Autodesk Inventor part; units mm, degrees
ref_plane "YZ Plane" through (0, 0, 0) normal (1, 0, 0) x (0, 1, 0)
ref_plane "XZ Plane" through (0, 0, 0) normal (0, 1, 0) x (-1, 0, 0)
ref_plane "XY Plane" through (0, 0, 0) normal (0, 0, 1) x (1, 0, 0)
sketch "Sketch1" plane through (0, 0, 0) normal (0, 1, 0) x (-1, 0, 0)
  line L0 (7.056, 3.3) -> (-24.7, 3.3)
  line L1 (-24.7, 3.3) -> (-24.7, 5.5)
  line L2 (-24.7, 5.5) -> (-20.7, 5.5)
  line L3 (-20.7, 5.5) -> (-20.2, 5)
  line L4 (-20.2, 5) -> (20.2, 5)
  line L5 (20.2, 5) -> (20.7, 5.5)
  line L6 (20.7, 5.5) -> (24.7, 5.5)
  line L7 (24.7, 5.5) -> (24.7, 3.3)
  line L8 (24.7, 3.3) -> (7.056, 3.3)
  line L9 (0, -1.1) -> (0, 6.6) construction
  line L10 (-34.58, 0) -> (34.58, 0) construction
  point P0 (0, 0)
  dimension "d0" = 3.3
  dimension "d1" = 40.4
  dimension "d2" = 49.4
  dimension "d3" = 0.5
  dimension "d4" = 5
revolve "Revolution1" add sketch "Sketch1" angle 360 about axis through (0, 0, 0) along (-1, 0, 0)
properties part number "roller_ext"
Could you check a few things on this model? Use its own coordinates, in mm. A direction names the side the tool comes from. Coordinates: 2 decimals unless noted, no trailing zeros. Write each loop counter-clockwise with the first axis right and the second up, starting at its lowest first coordinate (ties: lowest second). Pieces come first, ordered by that corner, then holes. Notation, with made-up numbers: (17.25, 75.25) -> (28.25, 75.25) arc R31 cw to (28.25, 102.25) -> close; hole circle Ø4 at (42, 20.5). An arc over 180 degrees is marked (long way). Write item = value, one per line. Start each with the question number.
(1) Will these pins go through, and if not, where does the flat tip stop? pin 1 (3 mm diameter, centred on x = -10, z = 3, fed in from -Y); pin 2 (4 mm diameter, centred on x = -8, y = -1.5, fed in from -Z).
(2) I want a section at D-D (x = 13.5). Please give me the cut outline in (y, z).
(3) I want a section at A-A (y = 0). Please give me the cut outline in (x, z), plus the area to 3 significant figures.
(4) I need wall thicknesses on line 1 (Y direction, x = -5, z = 0); line 2 (Z direction, x = 6.5, y = -3.75); line 3 (Y direction, x = 3, z = -2.25). Which ranges of each line are inside material? Lowest first, please. Write a range as [from, to].
(5) Which directions (+Z, -Z, +X, -X, +Y, -Y) give clear straight access to the entire face, cutting with the end or side of a thin tool? Please do faces 1 (the face through (-0.28, -4.88, -1.08)), 2 (the face through (-22.73, -5.37, -1.19)).
(6) We'd pull the mould along Y, two halves only. Please class faces 3 (the face through (24.7, 0, 4)), 4 (the face through (22.67, -5.37, -1.19)), 5 (the face through (0.35, -2.23, -2.43)): released by +Y, released by -Y, zero draft, split by the parting line, or undercut.
(7) I want a section at C-C (x = 21.5). Please give me the cut outline in (y, z), plus the area to 3 significant figures.
Result set:
q1.pin_1 = -4.77
q1.pin_2 = -5
q2.outline = circle Ø10 at (0, 0); hole circle Ø6.6 at (0, 0)
q3.outline = (-24.7, -5.5) -> (-20.7, -5.5) -> (-20.2, -5) -> (20.2, -5) -> (20.7, -5.5) -> (24.7, -5.5) -> (24.7, -3.3) -> (-24.7, -3.3) -> close; (-24.7, 3.3) -> (24.7, 3.3) -> (24.7, 5.5) -> (20.7, 5.5) -> (20.2, 5) -> (-20.2, 5) -> (-20.7, 5.5) -> (-24.7, 5.5) -> close
q3.area = 176 mm2
q4.line_1 = [-5, -3.3], [3.3, 5]
q4.line_2 = [-3.31, 3.31]
q4.line_3 = [-4.47, -2.41], [2.41, 4.47]
q5.face_1 = none
q5.face_2 = +X, -X
q6.face_3 = zero draft
q6.face_4 = split by the parting line
q6.face_5 = undercut
q7.outline = circle Ø11 at (0, 0); hole circle Ø6.6 at (0, 0)
q7.area = 60.8 mm2
